Source: CAD feature listing. Evaluate the final solid. Frame: model axes, mm. Round coordinates to 2 decimals unless told otherwise and drop trailing zeros. Order: outer loops, then holes, each group sorted by start corner. A loop starts at its lowest first (then second) coordinate and runs counter-clockwise, first axis right, second up.
```python
from build123d import *

# Parameters (mm, degrees)
BOSS_EXTRUDE1_DEPTH = 2.3622
CUT_EXTRUDE1_DEPTH  = 124.949730405


with BuildPart() as part:
    # Sketch1 → Boss-Extrude1 (new body)
    with BuildSketch(Plane.XY):
        Polygon((-77.381787364, 72.847015101), (-77.381787364, 55.177029121), (-79.743987364, 55.177029121), (-79.743987364, 35.177029121), (-77.381787364, 35.177029121), (-77.381787364, 0.437015101), (-79.743987364, 0.437015101), (-79.743987364, -19.562984899), (-77.381787364, -19.562984899), (-77.381787364, -39.562984899), (97.893812636, -39.562984899), (97.893812636, -19.562984899), (100.256012636, -19.562984899), (100.256012636, 0.437015101), (97.893812636, 0.437015101), (97.893812636, 35.177029121), (100.256012636, 35.177029121), (100.256012636, 55.177029121), (97.893812636, 55.177029121), (97.893812636, 72.847015101), align=None)
    extrude(amount=BOSS_EXTRUDE1_DEPTH)

    # Sketch2 → Cut-Extrude1 (cut, through all)
    with BuildSketch(Plane.XY.offset(2.3622)):
        with BuildLine():
            Line((-52.243987364, 22.847015101), (72.756012636, 22.847015101))
            ThreePointArc((72.756012636, 22.847015101), (75.756012636, 19.847015101), (72.756012636, 16.847015101))
            Line((72.756012636, 16.847015101), (-52.243987364, 16.847015101))
            ThreePointArc((-52.243987364, 16.847015101), (-55.243987364, 19.847015101), (-52.243987364, 22.847015101))
        make_face()
        with BuildLine():
            Line((-52.243987364, 10.847015101), (72.756012636, 10.847015101))
            ThreePointArc((72.756012636, 10.847015101), (75.756012636, 7.847015101), (72.756012636, 4.847015101))
            Line((72.756012636, 4.847015101), (-52.243987364, 4.847015101))
            ThreePointArc((-52.243987364, 4.847015101), (-55.243987364, 7.847015101), (-52.243987364, 10.847015101))
        make_face()
        with BuildLine():
            Line((-52.243987364, -1.152984899), (72.756012636, -1.152984899))
            ThreePointArc((72.756012636, -1.152984899), (75.756012636, -4.152984899), (72.756012636, -7.152984899))
            Line((72.756012636, -7.152984899), (-52.243987364, -7.152984899))
            ThreePointArc((-52.243987364, -7.152984899), (-55.243987364, -4.152984899), (-52.243987364, -1.152984899))
        make_face()
    extrude(amount=-CUT_EXTRUDE1_DEPTH, mode=Mode.SUBTRACT)


solid = part.part
```
1. First-contact query: pin 1 (1.2 mm diameter, centred on y = 61, z = 1.5, fed in from +X); pin 2 (0.7 mm diameter, centred on y = -28, z = 1.5, fed in from -X); pin 3 (1.2 mm diameter, centred on x = 99.5, z = 0.5, fed in from -Y). Flat tips, straight axial feed; report the tip coordinate or a pass-through.
2. Section A-A on x = 62. Return loops of the section in (y, z).
3. Section B-B on z = 1.75. State how many separate pieces and enclosed holes the cut face has, plus the area to 3 significant figures.
4. Line query: line 1 along Y through (x, z) = (-13.5, 1.9); line 2 along Y through (x, z) = (74.5, 2.2); line 3 along X through (y, z) = (64.5, 1.8). Output: solid intervals per line, ascending.
5. Section C-C on y = 63. Return loops of the section in (x, z), plus the area to 3 significant figures.
Result:
1. pin 1: stops at x = 97.89
1. pin 2: stops at x = -77.38
1. pin 3: stops at y = -19.56
2. outline: (-39.56, 0) - (-7.15, 0) - (-7.15, 2.36) - (-39.56, 2.36) - close; (-1.15, 0) - (4.85, 0) - (4.85, 2.36) - (-1.15, 2.36) - close; (10.85, 0) - (16.85, 0) - (16.85, 2.36) - (10.85, 2.36) - close; (22.85, 0) - (72.85, 0) - (72.85, 2.36) - (22.85, 2.36) - close
3. separate pieces: 1
3. enclosed holes: 3
3. area: 17,600 mm2
4. line 1: y = -39.56 to -7.15, -1.15 to 4.85, 10.85 to 16.85, 22.85 to 72.85
4. line 2: y = -39.56 to -6.59, -1.71 to 5.41, 10.29 to 17.41, 22.29 to 72.85
4. line 3: x = -77.38 to 97.89
5. outline: (-77.38, 0) - (97.89, 0) - (97.89, 2.36) - (-77.38, 2.36) - close
5. area: 414 mm2
